Design review of the part built by this model. Coordinates are the model's own, in mm. Coordinates: 2 decimals unless noted, no trailing zeros. Write each loop counter-clockwise with the first axis right and the second up, starting at its lowest first coordinate (ties: lowest second). Pieces come first, ordered by that corner, then holes. Notation, with made-up numbers: M 40,2 L 56,2 A27 ccw 56,29 Z; hole C 48.25,24 d3. An arc over 180 degrees is marked long. Write item = value, one per line.
```python
from build123d import *

# Parameters (mm, degrees)
SCHIZZO1_W                    = 115
SCHIZZO1_H                    = 160
SCHIZZO1_W_2                  = 98
SCHIZZO1_H_2                  = 40
ESTRUSIONE_ESTRUSIONE1_DEPTH  = 2
SCHIZZO2_R                    = 3.5
SCHIZZO2_R_2                  = 1.25
ESTRUSIONE_ESTRUSIONE2_DEPTH  = 7.5
SCHIZZO3_R                    = 2.5
SCHIZZO3_R_2                  = 1.25
ESTRUSIONE_ESTRUSIONE3_DEPTH  = 3.5
SCHIZZO4_W                    = 121
SCHIZZO4_H                    = 166
SCHIZZO4_W_2                  = 115
SCHIZZO4_H_2                  = 160
ESTRUSIONE_ESTRUSIONE4_DEPTH  = 15
SCHIZZO5_W                    = 117
SCHIZZO5_H                    = 162
SCHIZZO5_W_2                  = 115
SCHIZZO5_H_2                  = 160
ESTRUSIONE_ESTRUSIONE5_DEPTH  = 1
RACCORDO2_R                   = 5
RACCORDO3_R                   = 3
SCHIZZO6_W                    = 6
SCHIZZO6_H                    = 6
SCHIZZO6_R                    = 1.75
ESTRUSIONE_ESTRUSIONE6_DEPTH  = 14
SCHIZZO7_R                    = 2.5
SCHIZZO7_R_2                  = 1.25
ESTRUSIONE_ESTRUSIONE7_DEPTH  = 25
SCHIZZO8_W                    = 20
SCHIZZO8_H                    = 4
ESTRUSIONE_ESTRUSIONE8_DEPTH  = 20
SCHIZZO9_W                    = 5
SCHIZZO9_H                    = 15
ESTRUSIONE_ESTRUSIONE9_DEPTH  = 15
SMUSSO1_SIZE                  = 15
SCHIZZO10_R                   = 0.75
TAGLIO_ESTRUSIONE1_DEPTH      = 15
SCHIZZO11_R                   = 7.35
SCHIZZO11_R_2                 = 6.35
ESTRUSIONE_ESTRUSIONE10_DEPTH = 5
SCHIZZO12_W                   = 5
SCHIZZO12_H                   = 5
ESTRUSIONE_ESTRUSIONE11_DEPTH = 6
SCHIZZO13_R                   = 1.5
TAGLIO_ESTRUSIONE2_DEPTH      = 142.992957572


with BuildPart() as part:
    # Schizzo1 → Estrusione-Estrusione1 (new body)
    with BuildSketch(Plane.XY):
        Rectangle(SCHIZZO1_W, SCHIZZO1_H)
        with Locations((0, 45)):
            Rectangle(SCHIZZO1_W_2, SCHIZZO1_H_2, mode=Mode.SUBTRACT)
    extrude(amount=ESTRUSIONE_ESTRUSIONE1_DEPTH)

    # Schizzo2 → Estrusione-Estrusione2 (add)
    # profile 1 of 4: a face of its own
    with BuildSketch(Plane.XY.offset(2)):
        with Locations((-46.5, 72.5)):
            Circle(SCHIZZO2_R)
        with Locations((-46.5, 72.5)):
            Circle(SCHIZZO2_R_2, mode=Mode.SUBTRACT)
    # profile 2 of 4: a face of its own
    with BuildSketch(Plane.XY.offset(2)):
        with Locations((-46.5, 17.5)):
            Circle(SCHIZZO2_R)
        with Locations((-46.5, 17.5)):
            Circle(SCHIZZO2_R_2, mode=Mode.SUBTRACT)
    # profile 3 of 4: a face of its own
    with BuildSketch(Plane.XY.offset(2)):
        with Locations((46.5, 17.5)):
            Circle(SCHIZZO2_R)
        with Locations((46.5, 17.5)):
            Circle(SCHIZZO2_R_2, mode=Mode.SUBTRACT)
    # profile 4 of 4: a face of its own
    with BuildSketch(Plane.XY.offset(2)):
        with Locations((46.5, 72.5)):
            Circle(SCHIZZO2_R)
        with Locations((46.5, 72.5)):
            Circle(SCHIZZO2_R_2, mode=Mode.SUBTRACT)
    extrude(amount=ESTRUSIONE_ESTRUSIONE2_DEPTH)

    # Schizzo3 → Estrusione-Estrusione3 (add)
    # profile 1 of 4: a face of its own
    with BuildSketch(Plane.XY.offset(2)):
        with Locations((-13.25, 0)):
            Circle(SCHIZZO3_R)
        with Locations((-13.25, 0)):
            Circle(SCHIZZO3_R_2, mode=Mode.SUBTRACT)
    # profile 2 of 4: a face of its own
    with BuildSketch(Plane.XY.offset(2)):
        with Locations((13.25, 0)):
            Circle(SCHIZZO3_R)
        with Locations((13.25, 0)):
            Circle(SCHIZZO3_R_2, mode=Mode.SUBTRACT)
    # profile 3 of 4: a face of its own
    with BuildSketch(Plane.XY.offset(2)):
        with Locations((17.25, -38)):
            Circle(SCHIZZO3_R)
        with Locations((17.25, -38)):
            Circle(SCHIZZO3_R_2, mode=Mode.SUBTRACT)
    # profile 4 of 4: a face of its own
    with BuildSketch(Plane.XY.offset(2)):
        with Locations((-16.75, -38)):
            Circle(SCHIZZO3_R)
        with Locations((-16.75, -38)):
            Circle(SCHIZZO3_R_2, mode=Mode.SUBTRACT)
    extrude(amount=ESTRUSIONE_ESTRUSIONE3_DEPTH)

    # Schizzo4 → Estrusione-Estrusione4 (add)
    with BuildSketch(Plane(origin=(0, 0, 0), x_dir=(-1, 0, 0), z_dir=(0, 0, -1))):
        Rectangle(SCHIZZO4_W, SCHIZZO4_H)
        Rectangle(SCHIZZO4_W_2, SCHIZZO4_H_2, mode=Mode.SUBTRACT)
    extrude(amount=-ESTRUSIONE_ESTRUSIONE4_DEPTH)

    # Schizzo5 → Estrusione-Estrusione5 (add)
    with BuildSketch(Plane.XY.offset(15)):
        Rectangle(SCHIZZO5_W, SCHIZZO5_H)
        Rectangle(SCHIZZO5_W_2, SCHIZZO5_H_2, mode=Mode.SUBTRACT)
    extrude(amount=ESTRUSIONE_ESTRUSIONE5_DEPTH)

    # Raccordo2
    raccordo2_edges = [part.edges().sort_by_distance(p)[0] for p in [
        (60.5, 83, 7.5),
        (-60.5, 83, 7.5),
        (-60.5, -83, 7.5),
        (60.5, -83, 7.5),
    ]]
    fillet(raccordo2_edges, radius=RACCORDO2_R)

    # Raccordo3
    raccordo3_edges = [part.edges().sort_by_distance(p)[0] for p in [
        (-58.5, 81, 15.5),
        (-58.5, -81, 15.5),
        (58.5, -81, 15.5),
        (58.5, 81, 15.5),
    ]]
    fillet(raccordo3_edges, radius=RACCORDO3_R)

    # Schizzo6 → Estrusione-Estrusione6 (add)
    # profile 1 of 4: a face of its own
    with BuildSketch(Plane.XY.offset(2)):
        with Locations((-54.5, 77)):
            Rectangle(SCHIZZO6_W, SCHIZZO6_H)
        with Locations((-54.5, 77)):
            Circle(SCHIZZO6_R, mode=Mode.SUBTRACT)
    # profile 2 of 4: a face of its own
    with BuildSketch(Plane.XY.offset(2)):
        with Locations((54.5, 77)):
            Rectangle(SCHIZZO6_W, SCHIZZO6_H)
        with Locations((54.5, 77)):
            Circle(SCHIZZO6_R, mode=Mode.SUBTRACT)
    # profile 3 of 4: a face of its own
    with BuildSketch(Plane.XY.offset(2)):
        with Locations((-54.5, -77)):
            Rectangle(SCHIZZO6_W, SCHIZZO6_H)
        with Locations((-54.5, -77)):
            Circle(SCHIZZO6_R, mode=Mode.SUBTRACT)
    # profile 4 of 4: a face of its own
    with BuildSketch(Plane.XY.offset(2)):
        with Locations((54.5, -77)):
            Rectangle(SCHIZZO6_W, SCHIZZO6_H)
        with Locations((54.5, -77)):
            Circle(SCHIZZO6_R, mode=Mode.SUBTRACT)
    extrude(amount=ESTRUSIONE_ESTRUSIONE6_DEPTH)

    # Schizzo7 → Estrusione-Estrusione7 (add)
    # profile 1 of 4: a face of its own
    with BuildSketch(Plane.XY.offset(2)):
        with Locations((54.5, -5)):
            Circle(SCHIZZO7_R)
        with Locations((54.5, -5)):
            Circle(SCHIZZO7_R_2, mode=Mode.SUBTRACT)
    # profile 2 of 4: a face of its own
    with BuildSketch(Plane.XY.offset(2)):
        with Locations((31.5, -5)):
            Circle(SCHIZZO7_R)
        with Locations((31.5, -5)):
            Circle(SCHIZZO7_R_2, mode=Mode.SUBTRACT)
    # profile 3 of 4: a face of its own
    with BuildSketch(Plane.XY.offset(2)):
        with Locations((31.5, -63)):
            Circle(SCHIZZO7_R)
        with Locations((31.5, -63)):
            Circle(SCHIZZO7_R_2, mode=Mode.SUBTRACT)
    # profile 4 of 4: a face of its own
    with BuildSketch(Plane.XY.offset(2)):
        with Locations((54.5, -63)):
            Circle(SCHIZZO7_R)
        with Locations((54.5, -63)):
            Circle(SCHIZZO7_R_2, mode=Mode.SUBTRACT)
    extrude(amount=ESTRUSIONE_ESTRUSIONE7_DEPTH)

    # Schizzo8 → Estrusione-Estrusione8 (add)
    with BuildSketch(Plane.XY.offset(2)):
        with Locations((43, -5)):
            Rectangle(SCHIZZO8_W, SCHIZZO8_H)
        with Locations((43, -63)):
            Rectangle(SCHIZZO8_W, SCHIZZO8_H)
    extrude(amount=ESTRUSIONE_ESTRUSIONE8_DEPTH)

    # Schizzo9 → Estrusione-Estrusione9 (add)
    with BuildSketch(Plane.XY.offset(2)):
        with Locations((43, -14.5)):
            Rectangle(SCHIZZO9_W, SCHIZZO9_H)
        with Locations((43, -53.5)):
            Rectangle(SCHIZZO9_W, SCHIZZO9_H)
    extrude(amount=ESTRUSIONE_ESTRUSIONE9_DEPTH)

    # Smusso1
    smusso1_edges = [part.edges().sort_by_distance(p)[0] for p in [
        (43, -46, 17),
        (43, -22, 17),
    ]]
    chamfer(smusso1_edges, length=SMUSSO1_SIZE - 0.0001)  # a hair under: the kernel refuses the full size

    # Schizzo10 → Taglio-Estrusione1 (cut)
    with BuildSketch(Plane.XY.offset(2)):
        with Locations((0, -70)):
            Circle(SCHIZZO10_R)
    extrude(amount=-TAGLIO_ESTRUSIONE1_DEPTH, mode=Mode.SUBTRACT)

    # Schizzo11 → Estrusione-Estrusione10 (add)
    with BuildSketch(Plane.XY.offset(2)):
        with Locations((0, -70)):
            Circle(SCHIZZO11_R)
        with Locations((0, -70)):
            Circle(SCHIZZO11_R_2, mode=Mode.SUBTRACT)
    extrude(amount=ESTRUSIONE_ESTRUSIONE10_DEPTH)

    # Schizzo12 → Estrusione-Estrusione11 (add)
    with BuildSketch(Plane.XY.offset(2)):
        with Locations((-49, 2.5)):
            Rectangle(SCHIZZO12_W, SCHIZZO12_H)
    extrude(amount=ESTRUSIONE_ESTRUSIONE11_DEPTH)

    # Schizzo13 → Taglio-Estrusione2 (cut, through all)
    with BuildSketch(Plane.ZY.offset(51.5)):
        with Locations(Location((4.696636297, 2.763205457, 0), (0, 0, 270))):
            Circle(SCHIZZO13_R)
    extrude(amount=TAGLIO_ESTRUSIONE2_DEPTH, mode=Mode.SUBTRACT)


solid = part.part
```
Q1. Consider section A-A, the plane y = 44. State the section outline as (x, z) points, and give its area (3 significant figures).
Check result:
outline = M -60.5,0 L -49,0 L -49,2 L -57.5,2 L -57.5,16 L -58.5,16 L -58.5,15 L -60.5,15 Z; M 49,0 L 60.5,0 L 60.5,15 L 58.5,15 L 58.5,16 L 57.5,16 L 57.5,2 L 49,2 Z
area = 126 mm²
Q2. The part is to be moulded in two halves that separate along Y. For faces 1 (the flat face through (1, 83, 7)), 2 (the flat face through (-51.5, 2, 5)), 3 (the cylindrical face through (-52.883, 76.33, 8.902)), say which applies: +Y half, -Y half, draft (parallel to the pull), parting line (faces both ways), or undercut.
Check result:
face_1 = +Y half
face_2 = undercut
face_3 = undercut
Q3. Consider section C-C, the plane x = -37. State the section outline as (y, z) points, and give its area (3 significant figures).
Check result:
outline = M -83,0 L 25,0 L 25,2 L -80,2 L -80,16 L -81,16 L -81,15 L -83,15 Z; M 65,0 L 83,0 L 83,15 L 81,15 L 81,16 L 80,16 L 80,2 L 65,2 Z
area = 332 mm²
Q4. Consider section B-B, the plane z = 19. State the section outline as (x, y) points.
Check result:
outline = M 33,-65 L 53,-65 A2.5 ccw long 53,-61 L 33,-61 A2.5 ccw long Z; M 33,-7 L 53,-7 A2.5 ccw long 53,-3 L 33,-3 A2.5 ccw long Z; hole C 31.5,-63 d2.5; hole C 31.5,-5 d2.5; hole C 54.5,-63 d2.5; hole C 54.5,-5 d2.5
Q5. Consider section D-D, the plane y = 10. State the section outline as (x, z) points.
Check result:
outline = M -60.5,0 L 60.5,0 L 60.5,15 L 58.5,15 L 58.5,16 L 57.5,16 L 57.5,2 L -57.5,2 L -57.5,16 L -58.5,16 L -58.5,15 L -60.5,15 Z
Q6. For P1, Ø1.2, axis at x = 54, y = -5, coming from the +Z side; P2, Ø1.2, axis at x = 40, y = -5, coming from the +Z side; P3, Ø2, axis at x = 33, z = 18, coming from the +Y side, all flat-tipped, find the tip position at first contact; note any pin that passes through.
Check result:
P1 = 2
P2 = 22
P3 = -2.55
Q7. Wall thickness on line 1 (Y direction, x = 31.5, z = 13.25); line 2 (X direction, y = -10, z = 5.5); line 3 (Y direction, x = -54.5, z = 10): over which ranges is each line inside the solid? List them lowest first.
Check result:
line_1 = -83 to -80, -65.5 to -64.25, -61.75 to -60.5, -7.5 to -6.25, -3.75 to -2.5, 80 to 83
line_2 = -60.5 to -57.5, 40.5 to 45.5, 57.5 to 60.5
line_3 = -83 to -78.75, -75.25 to -74, 74 to 75.25, 78.75 to 83
